```python
from build123d import *
from build123d.topology import SkipClean

# Parameters (mm, degrees)
SKETCH_1_W           = 15
SKETCH_1_H           = 26
EXTRUDE_1_DEPTH      = 168
SKETCH_2_R           = 2.5
EXTRUDE_2_DEPTH      = 9
EXTRUDE_3_DEPTH      = 1
EXTRUDE_3_DEPTH_BACK = 19
SKETCH_3_R           = 3.5
SKETCH_3_R_2         = 2.5
SKETCH_4_W           = 85
SKETCH_4_H           = 21
CUT_EXTRUDE_1_DEPTH  = 24
CUT_EXTRUDE_2_DEPTH  = 33
SKETCH_6_W           = 78
SKETCH_6_H           = 21
CUT_EXTRUDE_3_DEPTH  = 33
SKETCH_7_W           = 15
SKETCH_7_H           = 59
EXTRUDE_4_DEPTH      = 26
SKETCH_8_R           = 2.5
CUT_EXTRUDE_4_DEPTH  = 23.5
SKETCH_9_R           = 2.5
EXTRUDE_5_DEPTH      = 2.5
EXTRUDE_START        = -2.5
SKETCH_10_R          = 2.5
EXTRUDE_6_DEPTH      = 2.5
SKETCH_11_R          = 3
CUT_EXTRUDE_5_DEPTH  = 82.5
SKETCH_12_W          = 56.5
SKETCH_12_H          = 21
CUT_EXTRUDE_6_DEPTH  = 82.5
SKETCH_13_W          = 15
SKETCH_13_H          = 59
CUT_EXTRUDE_7_DEPTH  = 23.5
SKETCH_14_W          = 15
SKETCH_14_H          = 21
CUT_EXTRUDE_8_DEPTH  = 23.5
EXTRUDE_START_2      = -23.5
EXTRUDE_7_DEPTH      = 23.5
FILLET_1_R           = 2
SKETCH_16_R          = 1.5
SKETCH_16_R_2        = 7
CUT_EXTRUDE_9_DEPTH  = 23.5
FILLET_2_R           = 1.5
FILLET_3_R           = 3


with BuildPart() as part:
    # 草图1 → 凸台-拉伸1 (new body)
    with BuildSketch(Plane.XY):
        with Locations((7.5, 13)):
            Rectangle(SKETCH_1_W, SKETCH_1_H)
    extrude(amount=EXTRUDE_1_DEPTH)

    # 草图2 → 凸台-拉伸2 (add, symmetric)
    with BuildSketch(Plane(origin=(0, 13, 0), x_dir=(1, 0, 0), z_dir=(0, 1, 0))):
        with BuildLine():
            Line((12.5, -183), (12.5, -168))
            Line((12.5, -168), (2.5, -168))
            Line((2.5, -168), (2.5, -183))
            ThreePointArc((2.5, -183), (7.5, -188), (12.5, -183))
        make_face()
        with Locations(Location((7.5, -183, 0), (0, 0, 180))):
            Circle(SKETCH_2_R, mode=Mode.SUBTRACT)
    extrude(amount=EXTRUDE_2_DEPTH, both=True)

    # 草图3 → 凸台-拉伸3 (add, two sides: drawn at the far end of the back side and taken through both)
    with BuildSketch(Plane(origin=(0, 22, 0), x_dir=(1, 0, 0), z_dir=(0, 1, 0)).offset(-EXTRUDE_3_DEPTH_BACK)):
        with Locations(Location((7.5, -183, 0), (0, 0, 180))):
            Circle(SKETCH_3_R)
        with Locations(Location((7.5, -183, 0), (0, 0, 180))):
            Circle(SKETCH_3_R_2, mode=Mode.SUBTRACT)
    extrude(amount=EXTRUDE_3_DEPTH + EXTRUDE_3_DEPTH_BACK)

    # 草图4 → 切除-拉伸1 (cut)
    with BuildSketch(Plane(origin=(15, 0, 0), x_dir=(0, 0, -1), z_dir=(1, 0, 0))):
        with Locations((-123, 13)):
            Rectangle(SKETCH_4_W, SKETCH_4_H)
    extrude(amount=-CUT_EXTRUDE_1_DEPTH, mode=Mode.SUBTRACT)

    # 草图5 → 切除-拉伸2 (cut)
    with BuildSketch(Plane(origin=(0, 26, 0), x_dir=(1, 0, 0), z_dir=(0, 1, 0))):
        with BuildLine():
            Line((6, 0), (9, 0))
            Line((9, 0), (9, -17))
            ThreePointArc((9, -17), (10.5, -18.5), (9, -20))
            Line((9, -20), (6, -20))
            ThreePointArc((6, -20), (4.5, -18.5), (6, -17))
            Line((6, -17), (6, 0))
        make_face()
    extrude(amount=-CUT_EXTRUDE_2_DEPTH, mode=Mode.SUBTRACT)

    # 草图6 → 切除-拉伸3 (cut)
    with BuildSketch(Plane(origin=(15, 0, 0), x_dir=(0, 0, -1), z_dir=(1, 0, 0))):
        with Locations((-39, 13)):
            Rectangle(SKETCH_6_W, SKETCH_6_H)
    extrude(amount=-CUT_EXTRUDE_3_DEPTH, mode=Mode.SUBTRACT)

    # 草图7 → 凸台-拉伸4 (add)
    with BuildSketch(Plane(origin=(0, 26, 0), x_dir=(1, 0, 0), z_dir=(0, 1, 0))):
        with Locations((22.5, -51)):
            Rectangle(SKETCH_7_W, SKETCH_7_H)
    extrude(amount=-EXTRUDE_4_DEPTH)

    # 草图8 → 切除-拉伸4 (cut)
    with BuildSketch(Plane(origin=(0, 26, 0), x_dir=(1, 0, 0), z_dir=(0, 1, 0))):
        with Locations(Location((12.5, -25.75, 0), (0, 0, 180))):
            Circle(SKETCH_8_R)
        with Locations(Location((22.5, -25.75, 0), (0, 0, 180))):
            Circle(SKETCH_8_R)
        with Locations(Location((12.5, -75.25, 0), (0, 0, 180))):
            Circle(SKETCH_8_R)
        with Locations(Location((22.5, -75.25, 0), (0, 0, 180))):
            Circle(SKETCH_8_R)
        with BuildLine():
            Line((10.5, -30.5), (24.5, -30.5))
            ThreePointArc((24.5, -30.5), (26, -29), (27.5, -30.5))
            Line((27.5, -30.5), (27.5, -70.5))
            ThreePointArc((27.5, -70.5), (26, -72), (24.5, -70.5))
            Line((24.5, -70.5), (10.5, -70.5))
            ThreePointArc((10.5, -70.5), (9, -72), (7.5, -70.5))
            Line((7.5, -70.5), (7.5, -30.5))
            ThreePointArc((7.5, -30.5), (9, -29), (10.5, -30.5))
        make_face()
    extrude(amount=-CUT_EXTRUDE_4_DEPTH, mode=Mode.SUBTRACT)

    # 草图9 → 凸台-拉伸5 (add)
    with SkipClean():  # the faces are left unmerged after this step: merging them gives an invalid solid
        with BuildSketch(Plane(origin=(0, 26, 0), x_dir=(1, 0, 0), z_dir=(0, 1, 0))):
            with BuildLine():
                Line((-4, -35.5), (1, -35.5))
                Line((1, -35.5), (1, -45.5))
                Line((1, -45.5), (-4, -45.5))
                ThreePointArc((-4, -45.5), (-9, -40.5), (-4, -35.5))
            make_face()
            with Locations(Location((-4, -40.5, 0), (0, 0, 180))):
                Circle(SKETCH_9_R, mode=Mode.SUBTRACT)
        extrude(amount=-EXTRUDE_5_DEPTH)

    # 草图10 → 凸台-拉伸6 (add)
    with SkipClean():  # the faces are left unmerged after this step: merging them gives an invalid solid
        with BuildSketch(Plane.XZ.offset(EXTRUDE_START)):
            with BuildLine():
                Line((-4, 45.5), (1, 45.5))
                Line((1, 45.5), (1, 35.5))
                Line((1, 35.5), (-4, 35.5))
                ThreePointArc((-4, 35.5), (-9, 40.5), (-4, 45.5))
            make_face()
            with Locations(Location((-4, 40.5, 0), (0, 0, 180))):
                Circle(SKETCH_10_R, mode=Mode.SUBTRACT)
        extrude(amount=EXTRUDE_6_DEPTH)

    # 草图11 → 切除-拉伸5 (cut)
    with SkipClean():  # the faces are left unmerged after this step: merging them gives an invalid solid
        with BuildSketch(Plane.XZ):
            with Locations(Location((7.5, 138, 0), (0, 0, 270))):
                Circle(SKETCH_11_R)
        extrude(amount=-CUT_EXTRUDE_5_DEPTH, mode=Mode.SUBTRACT)

    # 草图12 → 切除-拉伸6 (cut)
    with BuildSketch(Plane.ZY.offset(-15)):
        with Locations((49.75, 13)):
            Rectangle(SKETCH_12_W, SKETCH_12_H)
    extrude(amount=-CUT_EXTRUDE_6_DEPTH, mode=Mode.SUBTRACT)

    # 草图13 → 切除-拉伸7 (cut)
    with BuildSketch(Plane.XZ):
        with Locations((22.5, 51)):
            Rectangle(SKETCH_13_W, SKETCH_13_H)
    extrude(amount=-CUT_EXTRUDE_7_DEPTH, mode=Mode.SUBTRACT)

    # 草图14 → 切除-拉伸8 (cut)
    with BuildSketch(Plane(origin=(0, 0, 78), x_dir=(-1, 0, 0), z_dir=(0, 0, -1))):
        with Locations((-7.5, 13)):
            Rectangle(SKETCH_14_W, SKETCH_14_H)
    extrude(amount=-CUT_EXTRUDE_8_DEPTH, mode=Mode.SUBTRACT)

    # 草图15 → 凸台-拉伸7 (add)
    with BuildSketch(Plane.XZ.offset(EXTRUDE_START_2)):
        with BuildLine():
            Line((0, 20), (6, 20))
            ThreePointArc((6, 20), (4.5, 18.5), (6, 17))
            Line((6, 17), (6, 0))
            Line((6, 0), (0, 0))
            Line((0, 0), (0, 20))
        make_face()
        with BuildLine():
            Line((9, 20), (15, 20))
            Line((15, 20), (15, 0))
            Line((15, 0), (9, 0))
            Line((9, 0), (9, 17))
            ThreePointArc((9, 17), (10.5, 18.5), (9, 20))
        make_face()
    extrude(amount=EXTRUDE_7_DEPTH)

    # 圆角1
    # the kernel refuses this fillet: 2 mm, written as the material it adds along each edge
    with BuildSketch(Plane(origin=(15, 26, 80.5), x_dir=(1, 0, 0), z_dir=(0, -1, 0)), Plane(origin=(0, 26, 35.5), x_dir=(-1, 0, 0), z_dir=(0, -1, 0)), Plane(origin=(0, 23.5, 45.5), x_dir=(-1, 0, 0), z_dir=(0, 1, 0)), Plane(origin=(0, 2.5, 45.5), x_dir=(0, 0, 1), z_dir=(0, -1, 0))) as fillet_1_piece_1:
        with BuildLine():
            CenterArc((FILLET_1_R, FILLET_1_R), FILLET_1_R, 180, 90)
            Line((0, FILLET_1_R), (0, 0))
            Line((0, 0), (FILLET_1_R, 0))
        make_face()
    extrude(amount=2.5)
    with BuildSketch(Plane(origin=(15, 26, 21.5), x_dir=(1, 0, 0), z_dir=(0, -1, 0)), Plane(origin=(0, 0, 35.5), x_dir=(-1, 0, 0), z_dir=(0, 1, 0))) as fillet_1_piece_2:
        with BuildLine():
            CenterArc((FILLET_1_R, -FILLET_1_R), FILLET_1_R, 90, 90)
            Line((0, -FILLET_1_R), (0, 0))
            Line((0, 0), (FILLET_1_R, 0))
        make_face()
    extrude(amount=2.5)
    # the kernel refuses this fillet: 2 mm, written as the material it takes off along each edge
    with BuildSketch(Plane(origin=(30, 31, 21.5), x_dir=(-1, 0, 0), z_dir=(0, -1, 0)), Plane(origin=(30, 31, 80.5), x_dir=(0, 0, -1), z_dir=(0, -1, 0))) as fillet_1_2_piece_1:
        with BuildLine():
            CenterArc((FILLET_1_R, -FILLET_1_R), FILLET_1_R, 90, 90)
            Line((0, -FILLET_1_R), (0, 0))
            Line((0, 0), (FILLET_1_R, 0))
        make_face()
    extrude(amount=12.5, mode=Mode.SUBTRACT)

    # 草图16 → 切除-拉伸9 (cut)
    with BuildSketch(Plane.ZY):
        with Locations((4, 4)):
            Circle(SKETCH_16_R)
        with Locations((16, 4)):
            Circle(SKETCH_16_R)
        with Locations((4, 22)):
            Circle(SKETCH_16_R)
        with Locations((16, 22)):
            Circle(SKETCH_16_R)
        with Locations((10, 13)):
            Circle(SKETCH_16_R_2)
    extrude(amount=-CUT_EXTRUDE_9_DEPTH, mode=Mode.SUBTRACT)

    # 圆角2
    # the kernel refuses this fillet: 1.5 mm, written as the material it adds along each edge
    with BuildSketch(Plane(origin=(0, 23.5, 20), x_dir=(0, 0, 1), z_dir=(1, 0, 0)), Plane(origin=(5.25, 23.5, 20), x_dir=(0, 0, 1), z_dir=(1, 0, 0))) as fillet_2_piece_1:
        with BuildLine():
            CenterArc((FILLET_2_R, FILLET_2_R), FILLET_2_R, 180, 90)
            Line((0, FILLET_2_R), (0, 0))
            Line((0, 0), (FILLET_2_R, 0))
        make_face()
    extrude(amount=9.75)
    with BuildSketch(Plane(origin=(0, 2.5, 20), x_dir=(0, 0, 1), z_dir=(1, 0, 0)), Plane(origin=(5.25, 2.5, 20), x_dir=(0, 0, 1), z_dir=(1, 0, 0))) as fillet_2_piece_2:
        with BuildLine():
            CenterArc((FILLET_2_R, -FILLET_2_R), FILLET_2_R, 90, 90)
            Line((0, -FILLET_2_R), (0, 0))
            Line((0, 0), (FILLET_2_R, 0))
        make_face()
    extrude(amount=9.75)
    with BuildSketch(Plane(origin=(15, 2.5, 165.5), x_dir=(0, 1, 0), z_dir=(-1, 0, 0)), Plane(origin=(15, 23.5, 165.5), x_dir=(0, 0, -1), z_dir=(-1, 0, 0))) as fillet_2_piece_3:
        with BuildLine():
            CenterArc((FILLET_2_R, FILLET_2_R), FILLET_2_R, 180, 90)
            Line((0, FILLET_2_R), (0, 0))
            Line((0, 0), (FILLET_2_R, 0))
        make_face()
    extrude(amount=15)

    # 圆角3
    fillet_3_edges = [part.edges().sort_by_distance(p)[0] for p in [
        (12, 26, 0),
        (3, 0, 0),
        (3, 26, 0),
        (12, 0, 0),
    ]]
    fillet(fillet_3_edges, radius=FILLET_3_R)


solid = part.part
```
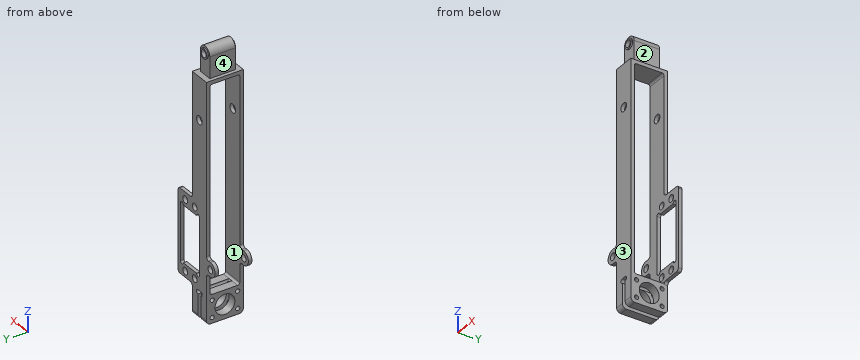
Work out the finished part from the listing and answer in its coordinate system (mm). Face numbers are marked on the shaded views. A direction names the side the tool comes from. Round coordinates to 2 decimals unless told otherwise and drop trailing zeros. Write each loop counter-clockwise with the first axis right and the second up, starting at its lowest first coordinate (ties: lowest second). Pieces come first, ordered by that corner, then holes.
1) A cutting plane is placed at B-B on x = 22.5. Determine the outline of the cut face in (y, z), and give its area (3 significant figures).
2) Which of the six approach directions +Z, -Z, +X, -X, +Y, -Y give full straight-line access (tool end or side, diameter ignored) to the marked faces 3 and 4?
3) A cutting plane is placed at D-D on z = 40.5. Determine the outline of the cut face in (x, y).
4) Flat-ended cylindrical pins translate along their axes: P1, Ø2.5, axis at y = 22, z = 16, coming from the +X side; P2, Ø3, axis at x = 20, y = 24.5, coming from the +Z side; P3, Ø4, axis at y = 4, z = 16, coming from the +X side; P4, Ø8, axis at x = 5.5, z = 182.5, coming from the +Y side. Find the tip coordinate at first contact, or state that the pin passes through.
5) A cutting plane is placed at A-A on z = 61.5. Determine the outline of the cut face in (x, y), and give its area (3 significant figures).
6) A cutting plane is placed at C-C on z = 107. Determine the outline of the cut face in (x, y).
7) Consider probe 1 along Z at (x, y) = (22.5, 24.1); probe 2 along Y at (x, z) = (1, 137.5); probe 3 along Z at (x, y) = (2, 7.5). Determine where each line is inside the solid, lowest interval first.
8) Determine the mould class of the marked faces 1 and 2 for opening direction Z: pulls with the +Z half, pulls with the -Z half, needs draft (parallel to the pull), parting line crosses it, or undercut.
Entries:
1. outline: (23.5, 21.5) - (26, 21.5) - (26, 23.25) - (23.5, 23.25) - close; (23.5, 28.25) - (26, 28.25) - (26, 30.5) - (23.5, 30.5) - close; (23.5, 70.5) - (26, 70.5) - (26, 72.75) - (23.5, 72.75) - close; (23.5, 77.75) - (26, 77.75) - (26, 80.5) - (23.5, 80.5) - close
1. area: 22.5 mm2
2. face 3: +Z, -Z, +X, -X, -Y
2. face 4: +Z, -X, +Y, -Y
3. outline: (-9, 0) - (-6.5, 0) - (-6.5, 2.5) - (-9, 2.5) - close; (-9, 23.5) - (-6.5, 23.5) - (-6.5, 26) - (-9, 26) - close; (-1.5, 0) - (15, 0) - (15, 2.5) - (-1.5, 2.5) - close; (-1.5, 23.5) - (7.5, 23.5) - (7.5, 26) - (-1.5, 26) - close; (27.5, 23.5) - (30, 23.5) - (30, 26) - (27.5, 26) - close
4. P1: passes through
4. P2: stops at z = 80.5
4. P3: stops at x = 15
4. P4: stops at y = 23
5. outline: (0, 0) - (15, 0) - (15, 2.5) - (0, 2.5) - close; (0, 23.5) - (7.5, 23.5) - (7.5, 26) - (0, 26) - close; (27.5, 23.5) - (30, 23.5) - (30, 26) - (27.5, 26) - close
5. area: 62.5 mm2
6. outline: (0, 0) - (15, 0) - (15, 2.5) - (0, 2.5) - close; (0, 23.5) - (15, 23.5) - (15, 26) - (0, 26) - close
7. probe 1: z = 21.5 to 23.25, 28.25 to 30.5, 70.5 to 72.75, 77.75 to 80.5
7. probe 2: y = 0 to 2.5, 23.5 to 26
7. probe 3: z = 0 to 5.67, 14.33 to 20, 165.5 to 168
8. face 1: undercut
8. face 2: needs draft
